CAD build for the part. Positions are in the model's coordinates, mm. A direction names the side the tool comes from. Round coordinates to 2 decimals unless told otherwise and drop trailing zeros. Write each loop counter-clockwise with the first axis right and the second up, starting at its lowest first coordinate (ties: lowest second). Pieces come first, ordered by that corner, then holes. Notation, with made-up numbers: (-6.5, 75.5) - (23.5, 75.5) arc R8 ccw to (23.5, 82.5) - close; hole circle Ø4 at (-34.5, -29.75). An arc over 180 degrees is marked (long way). Use one line per item in the form item = value. Start each with the question number.
Item 1: Band-saw the part on B-B, the plane y = 47. List the corners of the cut face in (x, z).
Item 2: Band-saw the part on D-D, the plane z = 4. Give the number of separate pieces and of enclosed holes in the cut face, and give its area (3 significant figures).
Item 3: Drill centre lines: L1, parallel to Y at x = 164, z = 3.75; L2, parallel to X at y = 8.5, z = 2; L3, parallel to Z at x = 213, y = 3. Where is each one in solid material? Low to high.
Item 4: Tool access for faces 5 (the flat face through (206.5, 20, 4)), 6 (the flat face through (0, 49, 4)), 7 (the flat face through (213, 8, 4)): list every direction of +Z, -Z, +X, -X, +Y, -Y with a clear straight run to the whole face (end or side of a thin tool).
Item 5: Band-saw the part on C-C, the plane y = 24. List the corners of the cut face in (x, z), and give its area (3 significant figures).
Item 6: Band-saw the part on A-A, the plane x = 56. List the corners of the cut face in (y, z), and give its area (3 significant figures).
Item 7: Pin check, flat tips, straight feed: pin 1 (2.5 mm diameter, centred on x = 33.5, z = 4, fed in from -Y); pin 2 (4 mm diameter, centred on y = 12.5, z = 4.5, fed in from -X); pin 3 (1.2 mm diameter, centred on x = 6, z = 3.5, fed in from -Y). Stop position of each tip, or through.
Item 8: Pull direction Z, two halves, no side cores. Call faces 1 (the cylindrical face through (210.79, 44.77, 3.94)), 2 (the flat face through (7, 8, 4)), 3 (the flat face through (108, 51, 0)), 4 (the flat face through (108, 51, 8)): +Z half, -Z half, draft (parallel to the pull), parting line (faces both ways), or undercut.
from build123d import *

# Parameters (mm, degrees)
ESQUISSE1_W                  = 220
ESQUISSE1_H                  = 100
BOSS_EXTRU_1_DEPTH           = 8
ESQUISSE2_R                  = 2
ENL_V_MAT_EXTRU_1_DEPTH      = 8
ENL_V_MAT_EXTRU_6_DEPTH      = 242.793300155
ENL_V_MAT_EXTRU_6_DEPTH_BACK = 242.793300155
ESQUISSE8_W                  = 32.5
ESQUISSE8_H                  = 40
ENL_V_MAT_EXTRU_8_DEPTH      = 242.793300155
ENL_V_MAT_EXTRU_8_DEPTH_BACK = 242.793300155
ESQUISSE10_R                 = 2.25


with BuildPart() as part:
    # Esquisse1 → Boss.-Extru.1 (new body)
    with BuildSketch(Plane.XY):
        with Locations((110, 50)):
            Rectangle(ESQUISSE1_W, ESQUISSE1_H)
    extrude(amount=BOSS_EXTRU_1_DEPTH)

    # Esquisse2 → Enlèv. mat.-Extru.1 (cut)
    with BuildSketch(Plane.XZ):
        with Locations(Location((110, 4, 0), (0, 0, 270))):
            Circle(ESQUISSE2_R)
        with Locations(Location((213, 4, 0), (0, 0, 270))):
            Circle(ESQUISSE2_R)
        with Locations(Location((7, 4, 0), (0, 0, 90))):
            Circle(ESQUISSE2_R)
    extrude(amount=-ENL_V_MAT_EXTRU_1_DEPTH, mode=Mode.SUBTRACT)

    # Esquisse8 → Enlèv. mat.-Extru.6 (cut, two sides: drawn at the far end of the back side and taken through both)
    with BuildSketch(Plane.XY.offset(8).offset(-ENL_V_MAT_EXTRU_6_DEPTH_BACK)):
        with Locations((190.25, 20)):
            Rectangle(ESQUISSE8_W, ESQUISSE8_H)
        with Locations((29.75, 20)):
            Rectangle(ESQUISSE8_W, ESQUISSE8_H)
    extrude(amount=ENL_V_MAT_EXTRU_6_DEPTH + ENL_V_MAT_EXTRU_6_DEPTH_BACK, mode=Mode.SUBTRACT)

    # Esquisse10 → Enlèv. mat.-Extru.8 (cut, two sides: drawn at the far end of the back side and taken through both)
    with BuildSketch(Plane.XY.offset(8).offset(-ENL_V_MAT_EXTRU_8_DEPTH_BACK)):
        with Locations((9.5, 12)):
            Circle(ESQUISSE10_R)
        with Locations((9.5, 47)):
            Circle(ESQUISSE10_R)
        with Locations(Location((210.5, 47, 0), (0, 0, 180))):
            Circle(ESQUISSE10_R)
        with Locations(Location((210.5, 12, 0), (0, 0, 180))):
            Circle(ESQUISSE10_R)
        with Locations(Location((56, 47, 0), (0, 0, 180))):
            Circle(ESQUISSE10_R)
        with Locations(Location((56, 12, 0), (0, 0, 180))):
            Circle(ESQUISSE10_R)
        with Locations((164, 12)):
            Circle(ESQUISSE10_R)
        with Locations((164, 47)):
            Circle(ESQUISSE10_R)
    extrude(amount=ENL_V_MAT_EXTRU_8_DEPTH + ENL_V_MAT_EXTRU_8_DEPTH_BACK, mode=Mode.SUBTRACT)


solid = part.part
Determined:
q1.outline = (0, 0) - (7.25, 0) - (7.25, 8) - (0, 8) - close; (11.75, 0) - (53.75, 0) - (53.75, 8) - (11.75, 8) - close; (58.25, 0) - (161.75, 0) - (161.75, 8) - (58.25, 8) - close; (166.25, 0) - (208.25, 0) - (208.25, 8) - (166.25, 8) - close; (212.75, 0) - (220, 0) - (220, 8) - (212.75, 8) - close
q2.separate_pieces = 1
q2.enclosed_holes = 8
q2.area = 19,200 mm²
q3.L1 = 0 to 9.75, 14.25 to 44.75, 49.25 to 100
q3.L2 = 0 to 13.5, 46 to 174, 206.5 to 220
q3.L3 = 0 to 2, 6 to 8
q4.face_5 = +Z, -Z, -Y
q4.face_6 = +Z, -Z, -X, +Y, -Y
q4.face_7 = -Y
q5.outline = (0, 0) - (13.5, 0) - (13.5, 8) - (0, 8) - close; (46, 0) - (174, 0) - (174, 8) - (46, 8) - close; (206.5, 0) - (220, 0) - (220, 8) - (206.5, 8) - close
q5.area = 1,240 mm²
q6.outline = (0, 0) - (9.75, 0) - (9.75, 8) - (0, 8) - close; (14.25, 0) - (44.75, 0) - (44.75, 8) - (14.25, 8) - close; (49.25, 0) - (100, 0) - (100, 8) - (49.25, 8) - close
q6.area = 728 mm²
q7.pin_1 = 40
q7.pin_2 = 0
q7.pin_3 = 8
q8.face_1 = draft
q8.face_2 = undercut
q8.face_3 = -Z half
q8.face_4 = +Z half
